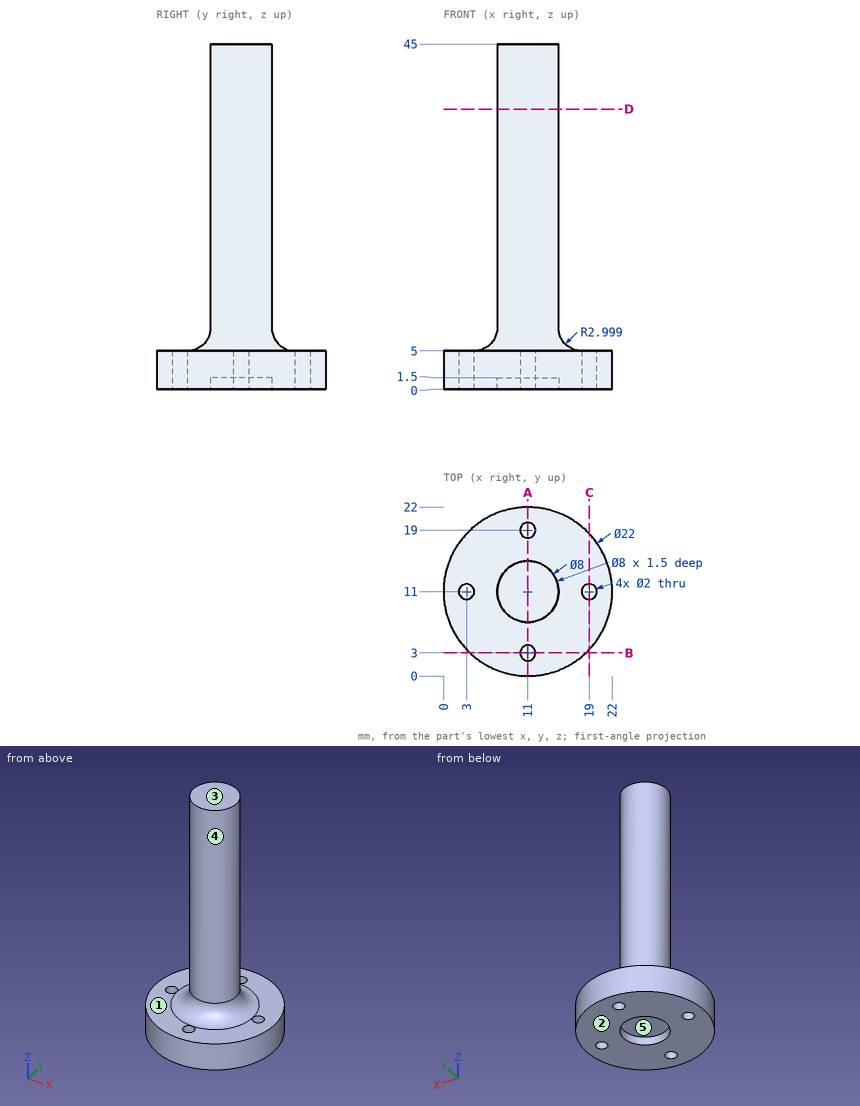
Could you check a few things on this drawing? It's one solid part, dimensions in mm from its lowest x, y, z. A direction names the side the tool comes from. Round coordinates to 2 decimals unless told otherwise and drop trailing zeros. Write each loop counter-clockwise with the first axis right and the second up, starting at its lowest first coordinate (ties: lowest second). Pieces come first, ordered by that corner, then holes.
Q1. If we mould it in two halves opening along X, with no side actions, what happens to the marked faces 3, 4 and 5? For each: +X half, -X half, draft (parallel to the pull), parting line (faces both ways), or undercut.
Q2. Which directions (+Z, -Z, +X, -X, +Y, -Y) give clear straight access to the entire face, cutting with the end or side of a thin tool? Please do the marked faces 1 and 2.
Q3. If we section it at B-B on y = 3: Write out the boundary of the cut face in (x, z), plus the area to 3 significant figures.
Q4. Please list where these lines run through material, in increasing order: probe 1 along Z at (x, y) = (2.25, 17.25); probe 2 along Z at (x, y) = (11, 10); probe 3 along Y at (x, z) = (3, 2).
Q5. Will these pins go through, and if not, where does the flat tip stop? P1, Ø1.5, axis at x = 14, y = 15, coming from the +Z side; P2, Ø6, axis at y = 15, z = 32, coming from the -X side; P3, Ø6, axis at x = 11, y = 3, coming from the +Z side (1 decimal); P4, Ø1.5, axis at x = 17, z = 31.5, coming from the -Y side.
Q6. If we section it at A-A on x = 11: Give the number of separate pieces and of enclosed holes in the cut face, plus the area to 3 significant figures.
Q7. If we section it at D-D on z = 36.5: Write out the boundary of the cut face in (x, y).
Answer below:
1. face 3: draft
1. face 4: parting line
1. face 5: undercut
2. face 1: +Z
2. face 2: -Z, +X, -X, +Y, -Y
3. outline: (3.45, 0) - (10, 0) - (10, 5) - (3.45, 5) - close; (12, 0) - (18.55, 0) - (18.55, 5) - (12, 5) - close
3. area: 65.5 mm2
4. probe 1: z = 0 to 5
4. probe 2: z = 1.5 to 45
4. probe 3: y = 3.45 to 10, 12 to 18.55
5. P1: stops at z = 6.8
5. P2: stops at x = 7.13
5. P3: stops at z = 5.8
5. P4: passes through
6. separate pieces: 3
6. enclosed holes: 0
6. area: 402 mm2
7. outline: circle Ø8 at (11, 11)
